CAD build for the part. Positions are in the model's coordinates, mm. A direction names the side the tool comes from. Coordinates: 2 decimals unless noted, no trailing zeros. Loops run counter-clockwise (first coordinate to the right, second up) from the corner with the lowest first, then second, coordinate; pieces in that order, holes last. Notation, with made-up numbers: (17.25, 7.25) - (43.25, 7.25) arc R26 ccw to (43.25, 46.25) - close; hole circle Ø9 at (-16, -26.5). An arc over 180 degrees is marked (long way). Put each result on its own line as item: value.
```python
from build123d import *

# Parameters (mm, degrees)
SKETCH_3_R      = 14.5
SKETCH_3_R_2    = 11
SKETCH_3_W      = 190
SKETCH_3_H      = 22
EXTRUDE_2_DEPTH = 3.5
SKETCH_5_R      = 14.5
SKETCH_5_R_2    = 13
EXTRUDE_3_DEPTH = 3.5


with BuildPart() as part:
    # Эскиз3 → Бобышка-Вытянуть2 (new body)
    with BuildSketch(Plane.XY):
        Circle(SKETCH_3_R)
        with Locations((-95, 0)):
            Circle(SKETCH_3_R_2)
        with Locations((95, 0)):
            Circle(SKETCH_3_R_2)
        Rectangle(SKETCH_3_W, SKETCH_3_H)
    extrude(amount=EXTRUDE_2_DEPTH)

    # Эскиз5 → Бобышка-Вытянуть3 (add)
    with BuildSketch(Plane.XY.offset(3.5)):
        Circle(SKETCH_5_R)
        Circle(SKETCH_5_R_2, mode=Mode.SUBTRACT)
    extrude(amount=EXTRUDE_3_DEPTH)


solid = part.part
```
Q1. Pin check, flat tips, straight feed: pin 1 Ø1.8 at (x, z) = (51.5, 1.5) entering from +Y; pin 2 Ø11 at (x, y) = (-46.5, 4.5) entering from +Z; pin 3 Ø3 at (x, z) = (73, 1) entering from -Y. Stop position of each tip, or through.
Determined:
pin 1: y = 11
pin 2: z = 3.5
pin 3: y = -11
Q2. Slice it at D-D, the plane x = 63.5. Give the cut face in (y, z), then the cut area to 3 significant figures.
Determined:
outline: (-11, 0) - (11, 0) - (11, 3.5) - (-11, 3.5) - close
area: 77.0 mm2
Q3. Slice it at C-C, the plane x = 0. Give the cut face in (y, z).
Determined:
outline: (-14.5, 0) - (14.5, 0) - (14.5, 7) - (13, 7) - (13, 3.5) - (-13, 3.5) - (-13, 7) - (-14.5, 7) - close
Q4. Wall check: L1, parallel to Y at x = 0, z = 4.45; L2, parallel to X at y = 0.75, z = 6.25; L3, parallel to Z at x = 43, y = 10.5. Give the ranges that are in metal, low to high. Write a range as from..to.
Determined:
L1: -14.5..-13, 13..14.5
L2: -14.48..-12.98, 12.98..14.48
L3: 0..3.5
Q5. Slice it at A-A, the plane z = 2. Give the cut face in (x, y), then the cut area to 3 significant figures.
Determined:
outline: (-95, -11) - (-9.45, -11) arc R14.5 ccw to (9.45, -11) - (95, -11) arc R11 ccw to (95, 11) - (9.45, 11) arc R14.5 ccw to (-9.45, 11) - (-95, 11) arc R11 ccw to start
area: 4,650 mm2
Q6. Slice it at B-B, the plane y = 0. Give the cut face in (x, z).
Determined:
outline: (-106, 0) - (106, 0) - (106, 3.5) - (14.5, 3.5) - (14.5, 7) - (13, 7) - (13, 3.5) - (-13, 3.5) - (-13, 7) - (-14.5, 7) - (-14.5, 3.5) - (-106, 3.5) - close
Q7. Mould opens along Y. For faces 1 (the cylindrical face through (-106, 0, 2)), 2 (the flat face through (0, 0, 3.5)), 3 (the flat face through (-58, 0, 3.5)) say: +Y half, -Y half, draft (parallel to the pull), parting line (faces both ways), or undercut.
Determined:
face 1: parting line
face 2: undercut
face 3: draft
Q8. Tool access for faces 4 (the flat face through (52, -11, 2)), 5 (the flat face through (-53, -11, 2)), 6 (the cylindrical face through (13.394, -5.554, 4.229)), 7 (the flat face through (-53, 11, 2)), 8 (the flat face through (52, 11, 2)): list every direction of +Z, -Z, +X, -X, +Y, -Y with a clear straight run to the whole face (end or side of a thin tool).
Determined:
face 4: +Z, -Z, +X, -Y
face 5: +Z, -Z, -X, -Y
face 6: +Z
face 7: +Z, -Z, -X, +Y
face 8: +Z, -Z, +X, +Y
